```python
from build123d import *

# Parameters (mm, degrees)
SKETCH1_W                 = 12.7
SKETCH1_H                 = 28.448
BOSS_EXTRUDE1_DEPTH       = 20.32
SKETCH2_W                 = 13.97
SKETCH2_H                 = 13.97
CUT_EXTRUDE1_DEPTH        = 28.866011125
SKETCH5_R                 = 1.5875
CUT_EXTRUDE2_DEPTH        = 36.531867443
F_4_40_TAPPED_HOLE1_D     = 2.2606
F_4_40_TAPPED_HOLE2_D     = 2.2606
F_4_40_TAPPED_HOLE2_DEPTH = 6.35
F_4_40_TAPPED_HOLE2_TIP   = 0.679152758
F_4_40_TAPPED_HOLE3_D     = 2.2606
F_4_40_TAPPED_HOLE3_DEPTH = 6.35
F_4_40_TAPPED_HOLE3_TIP   = 0.679152758


with BuildPart() as part:
    # Sketch1 → Boss-Extrude1 (new body)
    with BuildSketch(Plane(origin=(0, 0, 0), x_dir=(1, 0, 0), z_dir=(0, 1, 0))):
        Rectangle(SKETCH1_W, SKETCH1_H)
    extrude(amount=BOSS_EXTRUDE1_DEPTH)

    # Sketch2 → Cut-Extrude1 (cut, through all)
    with BuildSketch(Plane(origin=(6.35, 0, 0), x_dir=(0, 0, -1), z_dir=(1, 0, 0))):
        with Locations((0, 13.335)):
            Rectangle(SKETCH2_W, SKETCH2_H)
    extrude(amount=-CUT_EXTRUDE1_DEPTH, mode=Mode.SUBTRACT)

    # Sketch5 → Cut-Extrude2 (cut, through all)
    with BuildSketch(Plane.XY.offset(14.224)):
        with Locations((0, 17.145)):
            Circle(SKETCH5_R)
    extrude(amount=-CUT_EXTRUDE2_DEPTH, mode=Mode.SUBTRACT)

    # #4-40 Tapped Hole1 (through all)
    with Locations(Plane(origin=(0, 0, 0), x_dir=(-1, 0, 0), z_dir=(0, -1, 0))):
        with Locations((0, 0)):
            Hole(F_4_40_TAPPED_HOLE1_D / 2)

    # #4-40 Tapped Hole2
    with Locations(Plane(origin=(0, 0, -14.224), x_dir=(-1, 0, 0), z_dir=(0, 0, -1))):
        with Locations((0, 12.065), (0, 3.175)):
            Hole(F_4_40_TAPPED_HOLE2_D / 2, depth=F_4_40_TAPPED_HOLE2_DEPTH)
            with Locations((0, 0, -(F_4_40_TAPPED_HOLE2_DEPTH + F_4_40_TAPPED_HOLE2_TIP / 2))):  # 118° drill point
                Cone(0, F_4_40_TAPPED_HOLE2_D / 2, F_4_40_TAPPED_HOLE2_TIP, mode=Mode.SUBTRACT)

    # #4-40 Tapped Hole3
    with Locations(Plane.XY.offset(14.224)):
        with Locations((0, 12.065), (0, 3.175)):
            Hole(F_4_40_TAPPED_HOLE3_D / 2, depth=F_4_40_TAPPED_HOLE3_DEPTH)
            with Locations((0, 0, -(F_4_40_TAPPED_HOLE3_DEPTH + F_4_40_TAPPED_HOLE3_TIP / 2))):  # 118° drill point
                Cone(0, F_4_40_TAPPED_HOLE3_D / 2, F_4_40_TAPPED_HOLE3_TIP, mode=Mode.SUBTRACT)


solid = part.part
```
Geometry: final body of the model. Coordinates: model frame, mm. A direction names the side the tool comes from. Coordinates: 2 decimals unless noted, no trailing zeros. Write each loop counter-clockwise with the first axis right and the second up, starting at its lowest first coordinate (ties: lowest second). Pieces come first, ordered by that corner, then holes. Notation, with made-up numbers: M 51.25,-13.75 L 101.25,-13.75 A25 ccw 101.25,6.25 Z; hole C 56,77.5 d6. An arc over 180 degrees is marked long. Answer as CSV lines item,"result". Start each with the question number.
Q1. Reachability of faces 4 (the cylindrical face through (0.608, 4.128, -11.005)), 5 (the flat face through (0, 13, 6.985)), 6 (the cylindrical face through (0.147, 13.186, 11.005)) from +Z, -Z, +X, -X, +Y, -Y: full face, straight path, thin tool, end or side. Return the list, or none.
Q2. Mould query, pull axis Y, two halves, no side actions, for faces 1 (the flat face through (0, 20.32, -11)), 2 (the cylindrical face through (-0.245, 3.219, 1.103)), 3 (the conical face through (0.091, 3.001, 7.313)). Classes: released by +Y, released by -Y, zero draft, split by the parting line, or undercut.
Q3. Cut plane D-D on z = -9.75. Count the separate pieces of the cut face and the enclosed holes in it, then the cut area to 3 significant figures.
Q4. Cut plane B-B on x = 3.5. Return the cut outline in (y, z) (3 decimals).
Q5. Cut plane C-C on y = 9. Return the cut outline in (x, z) (3 decimals).
Q6. Line query: line 1 (Y direction, x = 0, z = 10); line 2 (Z direction, x = 3.75, y = 16.75) (3 decimals); line 3 (Y direction, x = 0.75, z = 13). Output: solid intervals per line, ascending. Write a range as from..to.
Q7. Cut plane A-A on z = 0. Return the cut outline in (x, y), then the cut area to 3 significant figures.
Q8. Pin query (flat end, axial travel): P1, Ø1, axis at x = 4, z = 0.5, coming from the +Y side; P2, Ø1.4, axis at x = 0, y = 3.175, coming from the +Z side. Return the tip coordinate at first contact, or that it passes through.
Findings below:
1,face 4,"-Z"
1,face 5,"+X, -X, +Y"
1,face 6,"+Z"
2,face 1,"released by +Y"
2,face 2,"zero draft"
2,face 3,"undercut"
3,separate pieces,"1"
3,enclosed holes,"3"
3,area,"242 mm2"
4,outline,"M 0,-14.224 L 20.32,-14.224 L 20.32,-6.985 L 6.35,-6.985 L 6.35,6.985 L 20.32,6.985 L 20.32,14.224 L 0,14.224 Z"
5,outline,"M -6.35,-14.224 L 6.35,-14.224 L 6.35,-6.985 L -6.35,-6.985 Z; M -6.35,6.985 L 6.35,6.985 L 6.35,14.224 L -6.35,14.224 Z"
6,line 1,"y = 0..2.04, 4.31..10.93, 13.2..15.56, 18.73..20.32"
6,line 2,"z = -14.224..-6.985, 6.985..14.224"
6,line 3,"y = 0..2.33, 4.02..11.22, 12.91..15.75, 18.54..20.32"
7,outline,"M -6.35,0 L -1.13,0 L -1.13,6.35 L -6.35,6.35 Z; M 1.13,0 L 6.35,0 L 6.35,6.35 L 1.13,6.35 Z"
7,area,"66.3 mm2"
8,P1,"stops at y = 6.35"
8,P2,"stops at z = 7.62"
